For this review, take the finished solid that the model builds, in its own axes (mm). Face numbers are marked on the shaded views. Give positions to 0.01 mm unless a question says otherwise; leave off trailing zeros. Write each loop counter-clockwise with the first axis right and the second up, starting at its lowest first coordinate (ties: lowest second). Pieces come first, ordered by that corner, then holes.
Q1. Mouldability with a two-part tool opening along X and no side actions: class the marked faces 1, 2, 3 and 4 as released by +X, released by -X, zero draft, split by the parting line, or undercut.
Q2. Insertion check: P1, Ø1.5, axis at x = -19.5, y = 3, coming from the +Z side; P2, Ø5, axis at x = 13.5, z = -0.5, coming from the +Y side; P3, Ø5, axis at x = 14.5, z = 0, coming from the -Y side; P4, Ø2.5, axis at y = 2.5, z = 0, coming from the -X side. Each pin has a flat end and moves straight along its axis. Give the tip position at first contact, or say it passes through.
Q3. We need section A-A (x = -17.5). Write out the cut boundary in (y, z), then the cut area to 3 significant figures.
Q4. For line 1 (Y direction, x = -21.1, z = 0); line 2 (X direction, y = 1.8, z = 0); line 3 (X direction, y = 2.25, z = -3.5), list the stretches that pass through material, from the lowest coordinate up.
```python
from build123d import *

# Parameters (mm, degrees)
SKETCH_2_W          = 43
SKETCH_2_H          = 14
EXTRUDE_1_DEPTH     = 5
SKETCH_6_R          = 5
CUT_EXTRUDE_4_DEPTH = 3.5
SKETCH_7_W          = 10
SKETCH_7_H          = 4.5
CUT_EXTRUDE_5_DEPTH = 10
FILLET_1_R          = 10
FILLET_2_R          = 10
FILLET_4_R          = 7
CHAMFER_1_SIZE      = 0.5
CHAMFER_1_SIZE2     = 0.181985117
FILLET_3_R          = 1
SKETCH_8_R          = 2.2
CUT_EXTRUDE_6_DEPTH = 3
FILLET_5_R          = 2
SKETCH_9_R          = 2
CUT_EXTRUDE_7_DEPTH = 4


# Some blends are built 0.0001 mm under size
with BuildPart() as part:
    # Эскиз2 → Бобышка-Вытянуть1 (new body)
    with BuildSketch(Plane(origin=(0, 0, 0), x_dir=(1, 0, 0), z_dir=(0, 1, 0))):
        Rectangle(SKETCH_2_W, SKETCH_2_H)
    extrude(amount=EXTRUDE_1_DEPTH)

    # Эскиз6 → Вырез-Вытянуть4 (cut)
    with BuildSketch(Plane(origin=(0, 5, 0), x_dir=(1, 0, 0), z_dir=(0, 1, 0))):
        with Locations(Location((14.5, 0, 0), (0, 0, 270))):
            Circle(SKETCH_6_R)
    extrude(amount=-CUT_EXTRUDE_4_DEPTH, mode=Mode.SUBTRACT)

    # Эскиз7 → Вырез-Вытянуть5 (cut)
    with BuildSketch(Plane(origin=(0, 5, 0), x_dir=(1, 0, 0), z_dir=(0, 1, 0))):
        with Locations((-16.5, -4.75)):
            Rectangle(SKETCH_7_W, SKETCH_7_H)
        with Locations((-16.5, 4.75)):
            Rectangle(SKETCH_7_W, SKETCH_7_H)
    extrude(amount=-CUT_EXTRUDE_5_DEPTH, mode=Mode.SUBTRACT)

    # Скругление1
    # the kernel refuses this fillet: 10 mm, written as the material it takes off along each edge
    with BuildSketch(Plane(origin=(-11.5, 25.879116361, 7), x_dir=(1, 0, 0), z_dir=(0, -1, 0))) as fillet_1_piece_1:
        with BuildLine():
            CenterArc((8.351646544, -10), FILLET_1_R, 90, 56.632987031)
            Line((0, -4.5), (-0.167032931, -4.39))
            ThreePointArc((-0.167032931, -4.39), (-0.2, -2.25), (-0.2, 0))
            Line((-0.2, 0), (0, 0.2))
            Line((0, 0.2), (8.351646544, 0.2))
            Line((8.351646544, 0.2), (8.351646544, 0))
        make_face()
    extrude(amount=46.758232721, mode=Mode.SUBTRACT)
    with BuildSketch(Plane(origin=(-11.5, 25.879116361, -7), x_dir=(1.535167055204576e-12, 0, 1.0), z_dir=(0, -1, 0))) as fillet_1_piece_2:
        with BuildLine():
            CenterArc((10, -8.351646544), FILLET_1_R, 123.367012969, 56.632987031)
            Line((0, -8.351646544), (-0.2, -8.351646544))
            Line((-0.2, -8.351646544), (-0.2, 0))
            Line((-0.2, 0), (0, 0.2))
            ThreePointArc((0, 0.2), (2.25, 0.2), (4.39, 0.167032931))
            Line((4.39, 0.167032931), (4.5, 0))
        make_face()
    extrude(amount=46.758232721, mode=Mode.SUBTRACT)

    # Скругление2
    fillet_2_edges = [part.edges().sort_by_distance(p)[0] for p in [
        (-11.5, 2.5, -2.5),
        (-11.5, 2.5, 2.5),
    ]]
    fillet(fillet_2_edges, radius=FILLET_2_R)

    # Скругление4
    fillet_4_edges = [part.edges().sort_by_distance(p)[0] for p in [
        (21.5, 2.5, -7),
        (21.5, 2.5, 7),
    ]]
    fillet(fillet_4_edges, radius=FILLET_4_R - 0.0001)  # a hair under: the kernel refuses the full size

    # Фаска1
    chamfer_1_edges = [part.edges().sort_by_distance(p)[0] for p in [
        (14.5, 5, -5),
    ]]
    chamfer_1_side = [part.faces().sort_by_distance(p)[0] for p in [
        (0.230514486, 5, 0),
    ]]
    chamfer(chamfer_1_edges, length=CHAMFER_1_SIZE, length2=CHAMFER_1_SIZE2, reference=chamfer_1_side[0])

    # Скругление3
    fillet_3_edges = [part.edges().sort_by_distance(p)[0] for p in [
        (-18.643789058, 0, 2.5),
        (-18.643789058, 5, -2.5),
        (5.675873272, 5, 7),
        (-6.502455422, 5, -6.420721841),
        (5.675873272, 0, 7),
        (-6.502455422, 0, 6.420721841),
        (-6.502455422, 0, -6.420721841),
        (-18.643789058, 0, -2.5),
        (-18.643789058, 5, 2.5),
        (-6.502455422, 5, 6.420721841),
        (-12.433476149, 5, -3.079278159),
        (-12.433476149, 0, -3.079278159),
        (-12.433476149, 5, 3.079278159),
        (-12.433476149, 0, 3.079278159),
        (5.675873272, 0, -7),
        (5.675873272, 5, -7),
        (19.449776758, 0, 4.949776758),
        (19.449776758, 0, -4.949776758),
        (19.449776758, 5, 4.949776758),
        (19.449776758, 5, -4.949776758),
    ]]
    fillet(fillet_3_edges, radius=FILLET_3_R)

    # Эскиз8 → Вырез-Вытянуть6 (cut)
    with BuildSketch(Plane.ZY.offset(21.5)):
        with Locations((0, 2.5)):
            Circle(SKETCH_8_R)
    extrude(amount=-CUT_EXTRUDE_6_DEPTH, mode=Mode.SUBTRACT)

    # Скругление5
    fillet_5_edges = [part.edges().sort_by_distance(p)[0] for p in [
        (-18.5, 2.5, -2.2),
    ]]
    fillet(fillet_5_edges, radius=FILLET_5_R)

    # Эскиз9 → Вырез-Вытянуть7 (cut)
    with BuildSketch(Plane(origin=(0, 1.5, 0), x_dir=(1, 0, 0), z_dir=(0, 1, 0))):
        with Locations(Location((14.5, 0, 0), (0, 0, 270))):
            Circle(SKETCH_9_R)
    extrude(amount=-CUT_EXTRUDE_7_DEPTH, mode=Mode.SUBTRACT)


solid = part.part
```
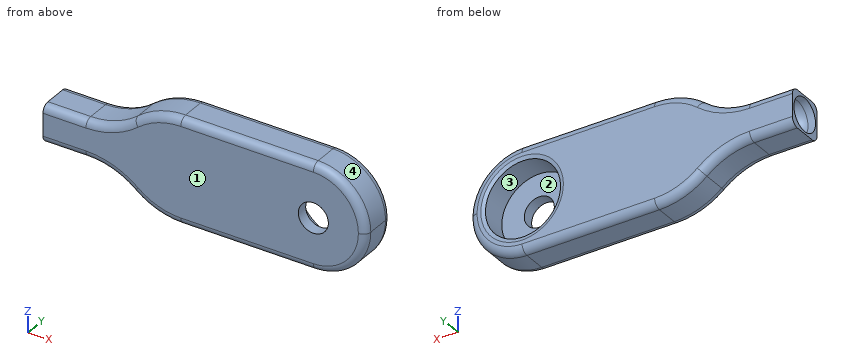
Computed:
1. face 1: zero draft
1. face 2: undercut
1. face 3: undercut
1. face 4: released by +X
2. P1: stops at z = 2.5
2. P2: stops at y = 1.5
2. P3: stops at y = 0
2. P4: stops at x = -18.8
3. outline: (0, -1.5) arc R1 ccw to (1, -2.5) - (4, -2.5) arc R1 ccw to (5, -1.5) - (5, 1.5) arc R1 ccw to (4, 2.5) - (1, 2.5) arc R1 ccw to (0, 1.5) - close
3. area: 24.1 mm2
4. line 1: y = 0 to 0.3, 4.7 to 5
4. line 2: x = -18.56 to 9.5, 19.5 to 21.5
4. line 3: x = -11.43 to 10.93, 18.07 to 20.56
